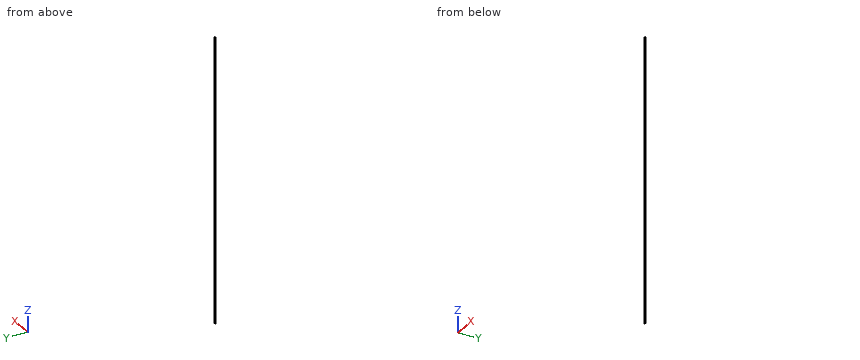
Autodesk Inventor part; units mm, degrees
ref_plane "Plano de trabajo1" through (-8.6166, 33.1799, 0) normal (-1, 0, 0) x (0, 0, -1)
ref_plane "Plano de trabajo2" through (0, 0, -993.7) normal (0, 0, 1) x (1, 0, 0)
ref_plane "YZ Plane" through (0, 0, 0) normal (1, 0, 0) x (0, 1, 0)
sketch "Boceto1" plane through (0, 0, 0) normal (0, 0, 1) x (1, 0, 0)
  line L0 (-13.5546, 31.7799) -> (-18.7766, 31.7799)
  line L1 (-12.1166, 33.1799) -> (-12.1166, 30.6799)
  line L2 (-12.1166, 30.6799) -> (-12.8266, 30.6799)
  line L3 (-12.8266, 30.6799) -> (-13.5546, 31.7799)
  arc A0 (-18.7766, 31.7799) -> (-21.5166, 29.0399) centre (-18.7766, 29.0399) ccw
  line L4 (-12.1166, 33.1799) -> (-8.6166, 33.1799)
  line L5 (-21.5166, 29.0399) -> (-21.5166, 26.2799)
  arc A1 (-8.6166, 33.1799) -> (-8.6166, 26.2799) centre (6.7872, 29.7299) ccw
  line L6 (-21.5166, 26.2799) -> (-21.0166, 26.2799)
  line L7 (-8.6166, 26.2799) -> (-9.1166, 26.2799)
  line L8 (-8.6166, 38.7215) -> (-8.6166, 22.0906) construction
  arc A2 (-9.1166, 26.2799) -> (-21.0166, 26.2799) centre (-15.0666, 20.0463) ccw
  dimension "d218" = 2.5
  dimension "d219" = 0.71
  dimension "d221" = 33.5
  dimension "d223" = 2.74
  dimension "d281" = 3.5
  dimension "d288" = 2.76
  dimension "d291" = 0.5
  dimension "d292" = 0.5
  dimension "d301" = 5.2219
extrude "Extrusión1" add sketch "Boceto1" against normal blind 1987.4
ref_plane "Plano de trabajo1" through (-8.6166, 33.1799, 0) normal (-1, 0, 0) x (0, 0, -1)
ref_plane "Plano de trabajo2" through (0, 0, -993.7) normal (0, 0, 1) x (1, 0, 0)
sketch "Boceto2" plane through (-8.6166, 33.1799, 0) normal (-1, 0, 0) x (0, 0, -1)
  line L0 (0, 0) -> (0, 6.9)
  line L1 (0, 0) -> (1987.4, 0)
  line L2 (6.9, 0) -> (0, 0)
  line L3 (0, 0) -> (0, 6.9)
  line L4 (0, 6.9) -> (1987.4, 6.9)
  line L5 (0, 6.9) -> (6.9, 0)
  point P0 (0, 0)
  dimension "d300" = 45
extrude "Extrusión2" cut sketch "Boceto2" along normal through all
properties part number "SP40-02 JUNTA INT CRISTAL 1987ç mm" material "Caucho"
Part model, mm, in its own coordinate system. Give positions to 0.01 mm unless a question says otherwise; leave off trailing zeros. Order: outer loops, then holes, each group sorted by start corner. A loop starts at its lowest first (then second) coordinate and runs counter-clockwise, first axis right, second up. Notation, with made-up numbers: (37.5, -16) - (50.5, -16) arc R13 cw to (50.5, 6) - close; hole circle Ø10 at (23.5, 88.25). An arc over 180 degrees is marked (long way). One line per question, with ' | ' between items.
1. Band-saw the part on A-A on z = -1734.5. List the corners of the cut face in (x, y).
Filled in:
outline: (-21.52, 26.28) - (-21.02, 26.28) arc R8.62 cw to (-9.12, 26.28) - (-8.62, 26.28) arc R15.79 cw to (-8.62, 33.18) - (-12.12, 33.18) - (-12.12, 30.68) - (-12.83, 30.68) - (-13.55, 31.78) - (-18.78, 31.78) arc R2.74 ccw to (-21.52, 29.04) - close
2. Band-saw the part on B-B on x = -15.75. List the corners of the cut face in (y, z).
Filled in:
outline: (28.64, -1987.4) - (31.78, -1987.4) - (31.78, -5.5) - (28.64, -2.36) - close
3. Drill centre lines: probe 1 along X at (y, z) = (28, -376); probe 2 along X at (y, z) = (30.75, -1217.5); probe 3 along Y at (x, z) = (-15.5, -1699). Where is each one in solid material? Low to high.
Filled in:
probe 1: -21.52 to -18.38, -11.75 to -8.9 | probe 2: -20.92 to -12.87, -12.12 to -8.97 | probe 3: 28.65 to 31.78
4. Drop flat-ended pins along their axis: P1, Ø5, axis at x = -17.5, z = -1271, coming from the -Y side; P2, Ø2, axis at x = -17.5, z = -1601.5, coming from the -Y side; P3, Ø1.5, axis at x = -16.5, y = 28, coming from the +Z side. Give the stop position or say it passes through.
Filled in:
P1: y = 27.11 | P2: y = 27.95 | P3: z = -2.13
